The listing builds one solid part. Answer for the finished solid, in the listing's coordinates (mm). Face numbers are marked on the shaded views. Coordinates: 2 decimals unless noted, no trailing zeros. Loops run counter-clockwise (first coordinate to the right, second up) from the corner with the lowest first, then second, coordinate; pieces in that order, holes last. Notation, with made-up numbers: (-37, 77.5) - (-2, 77.5) arc R15 cw to (-2, 86.5) - close; hole circle Ø2 at (18.5, 58.5). An arc over 180 degrees is marked (long way). Write each question's results on one line, items separated by ' | '. Start each with the question number.
(1) Given pin 1 Ø6 at (x, z) = (139.5, 71) entering from -Y; pin 2 Ø6 at (x, z) = (140.5, -46) entering from -Y; pin 3 Ø8 at (x, z) = (51.5, -35) entering from -Y, each flat-ended and moving along its own axis, determine where each tip first touches the part or whether it passes through.
(2) Consider line 1 (Y direction, x = 190, z = 2); line 2 (Y direction, x = 48, z = 23.5); line 3 (Z direction, x = 19, y = 27). Determine where each line is inside the solid, lowest interval first. Write a range as from..to.
(3) Find section D-D on y = 28.5. Determine the outline of the cut face in (x, z), then the cut area to 3 significant figures.
(4) Find section B-B on x = 147. Determine the outline of the cut face in (y, z), then the cut area to 3 significant figures.
(5) Find section A-A on z = 45. Determine the outline of the cut face in (x, y), then the cut area to 3 significant figures.
(6) Determine the mould class of the marked faces 1 and 2 for opening direction Z: released by +Z, released by -Z, zero draft, split by the parting line, or undercut.
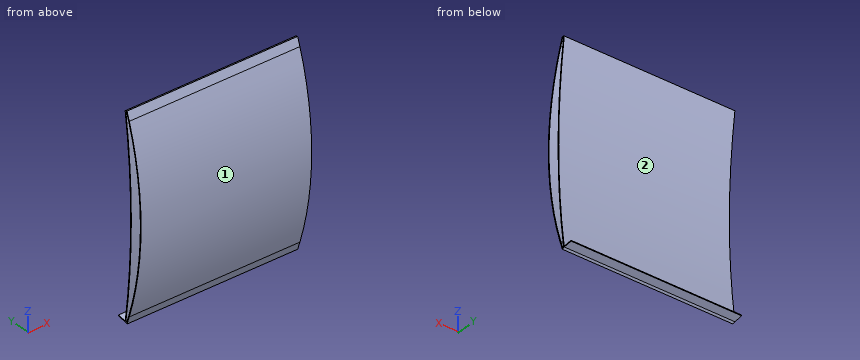
Autodesk Inventor part; units mm, degrees
ref_plane "YZ Plane" through (0, 0, 0) normal (1, 0, 0) x (0, 1, 0)
ref_plane "XZ Plane" through (0, 0, 0) normal (0, 1, 0) x (-1, 0, 0)
ref_plane "XY Plane" through (0, 0, 0) normal (0, 0, 1) x (1, 0, 0)
sketch "スケッチ1" plane through (0, 0, 0) normal (1, 0, 0) x (0, 1, 0)
  arc A0 (20.4585, 116.0261) -> (20.4585, -116.0261) centre (339.2375, 0) ccw
  line L0 (23.2776, 115) -> (20.4585, 116.0261)
  line L1 (23.2776, -115) -> (20.4585, -116.0261)
  line L2 (0, -162.4365) -> (0, 162.4365)
  arc A1 (23.2776, 115) -> (23.2776, -115) centre (836.8483, 0) ccw
  point P0 (0, 0)
  point P1 (0, 0)
  dimension "d0" = 3
  dimension "d1" = 230
  dimension "d2" = 40
  dimension "d12" = 3
extrude "押し出し1" add sketch "スケッチ1" along normal blind 200
sketch "スケッチ2" plane through (0, 0, 0) normal (-1, 0, 0) x (0, 0, 1)
  line L0 (-116.0261, 20.4585) -> (-106.5797, 17.1772)
  arc A0 (-116.0261, 20.4585) -> (116.0261, 20.4585) centre (0, 339.2375) ccw
  line L1 (0, 0) -> (0, -168.7214)
  line L2 (116.0261, 20.4585) -> (106.5797, 17.1772)
  arc A1 (-116.0261, 20.4585) -> (116.0261, 20.4585) centre (0, 339.2375) ccw
  point P0 (-116.0261, 20.4585)
  dimension "d13" = 10
extrude "押し出し2" cut sketch "スケッチ2" against normal through all
shell "シェル1" thickness 1 removed faces 2 at (0, 10.498, -16.8297) at (200, 10.498, -16.8297)
sketch "スケッチ6" plane through (200, 0, 0) normal (1, 0, 0) x (0, 0, -1)
  arc A0 (-115, 23.2776) -> (115, 23.2776) centre (0, 836.8483) ccw
  line L0 (115, 23.2776) -> (113.6004, 33.1792)
  line L1 (113.6004, 33.1792) -> (112.6102, 33.0392)
  line L2 (112.6102, 33.0392) -> (114.0098, 23.1382)
  point P0 (0, 0)
  dimension "d18" = 1
  dimension "d19" = 10
extrude "押し出し5" add sketch "スケッチ6" against normal blind 200
properties part number "element_gurnee" material "CFRP"
Values:
1) pin 1: stops at y = 6.89 | pin 2: stops at y = 2.74 | pin 3: stops at y = 1.42
2) line 1: y = 0.01..1.01, 14.19..15.19 | line 2: y = 0.81..1.82, 14.53..15.53 | line 3: z = -114.47..-113.46
3) outline: (0, -114.26) - (200, -114.26) - (200, -113.25) - (0, -113.25) - close | area: 202 mm²
4) outline: (17.18, -106.58) - (20.46, -116.03) - (23.28, -115) - (33.18, -113.6) - (33.04, -112.61) - (23.14, -114.01) arc R821.66 cw to (23.28, 115) - (20.46, 116.03) - (17.18, 106.58) arc R339.24 ccw to start; hole (18.12, -106.26) - (21.07, -114.74) - (22.17, -114.34) arc R822.66 cw to (22.17, 114.34) - (21.07, 114.74) - (18.12, 106.26) arc R338.24 ccw to start | area: 480 mm²
5) outline: (0, 3) - (200, 3) - (200, 4.01) - (0, 4.01) - close; (0, 15.42) - (200, 15.42) - (200, 16.42) - (0, 16.42) - close | area: 402 mm²
6) face 1: split by the parting line | face 2: undercut
